The figure shows three views and two pictorial views of one solid part (mm, origin at its lowest corner). Answer the questions. A direction names the side the tool comes from. Coordinates: 2 decimals unless noted, no trailing zeros. Loops run counter-clockwise (first coordinate to the right, second up) from the corner with the lowest first, then second, coordinate; pieces in that order, holes last. Notation, with made-up numbers: (28, -9) -> (40, -9) arc R29 ccw to (40, 30) -> close; hole circle Ø8 at (17.5, 89). An arc over 180 degrees is marked (long way). Answer as a JSON object with one key per item and string values. Group by question number.
1) Determine the mould class of the marked faces 1, 2, 3 and 4 for opening direction X: released by +X, released by -X, zero draft, split by the parting line, or undercut.
2) Section A-A, the plane x = 13 is taken. Give the vertices of the cut face in (y, z).
3) Which of the six approach directions +Z, -Z, +X, -X, +Y, -Y give full straight-line access (tool end or side, diameter ignored) to the marked faces 5, 6 and 7?
4) Consider probe 1 along Y at (x, z) = (13, 1.05); probe 2 along X at (y, z) = (8.5, 2.35); probe 3 along Y at (x, z) = (3.25, 1.1). Determine where each line is inside the solid, lowest interval first. Write a range as [from, to].
5) Section B-B, the plane y = 9 is taken. Give the vertices of the cut face in (x, z) (1 decimal).
6) Section D-D, the plane x = 7.5 is taken. Give the vertices of the cut face in (y, z), plus the area to 3 significant figures.
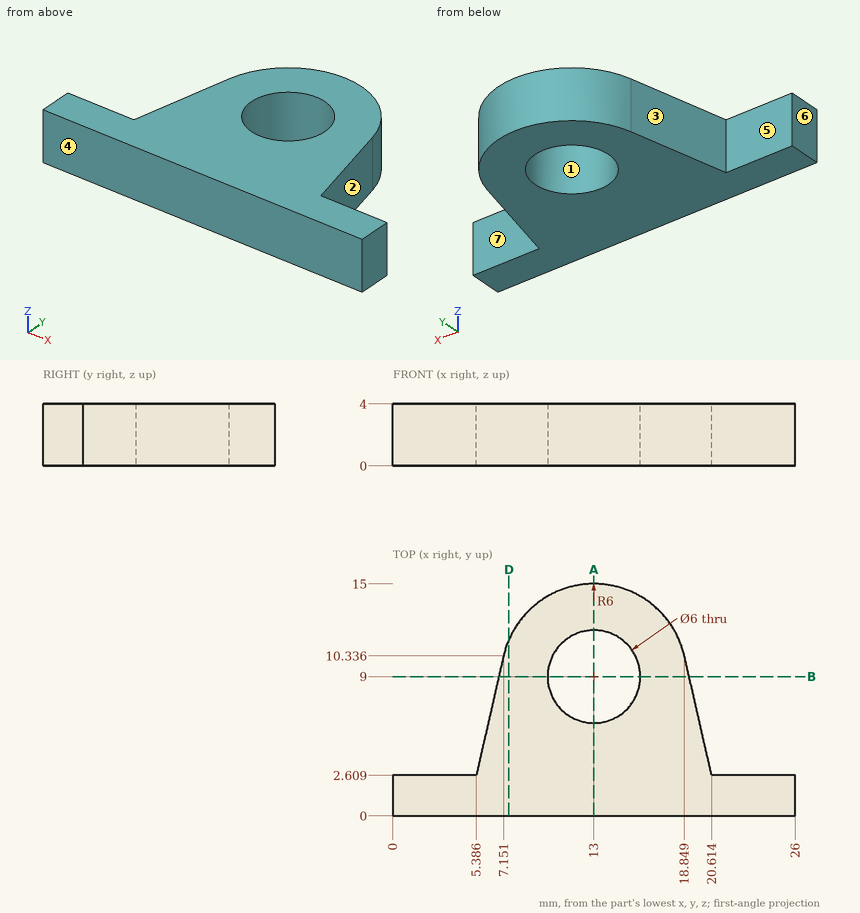
Determined:
{
 "1": {"face 1": "undercut", "face 2": "released by +X", "face 3": "released by -X", "face 4": "zero draft"},
 "2": {"outline": "(0, 0) -> (6, 0) -> (6, 4) -> (0, 4) -> close; (12, 0) -> (15, 0) -> (15, 4) -> (12, 4) -> close"},
 "3": {"face 5": "+Z, -Z, -X, +Y", "face 6": "+Z, -Z, -X, +Y, -Y", "face 7": "+Z, -Z, +X, +Y"},
 "4": {"probe 1": "[0, 6], [12, 15]", "probe 2": "[6.73, 10.04], [15.96, 19.27]", "probe 3": "[0, 2.61]"},
 "5": {"outline": "(6.8, 0) -> (10, 0) -> (10, 4) -> (6.8, 4) -> close; (16, 0) -> (19.2, 0) -> (19.2, 4) -> (16, 4) -> close"},
 "6": {"outline": "(0, 0) -> (11.4, 0) -> (11.4, 4) -> (0, 4) -> close", "area": "45.6 mm²"}
}
